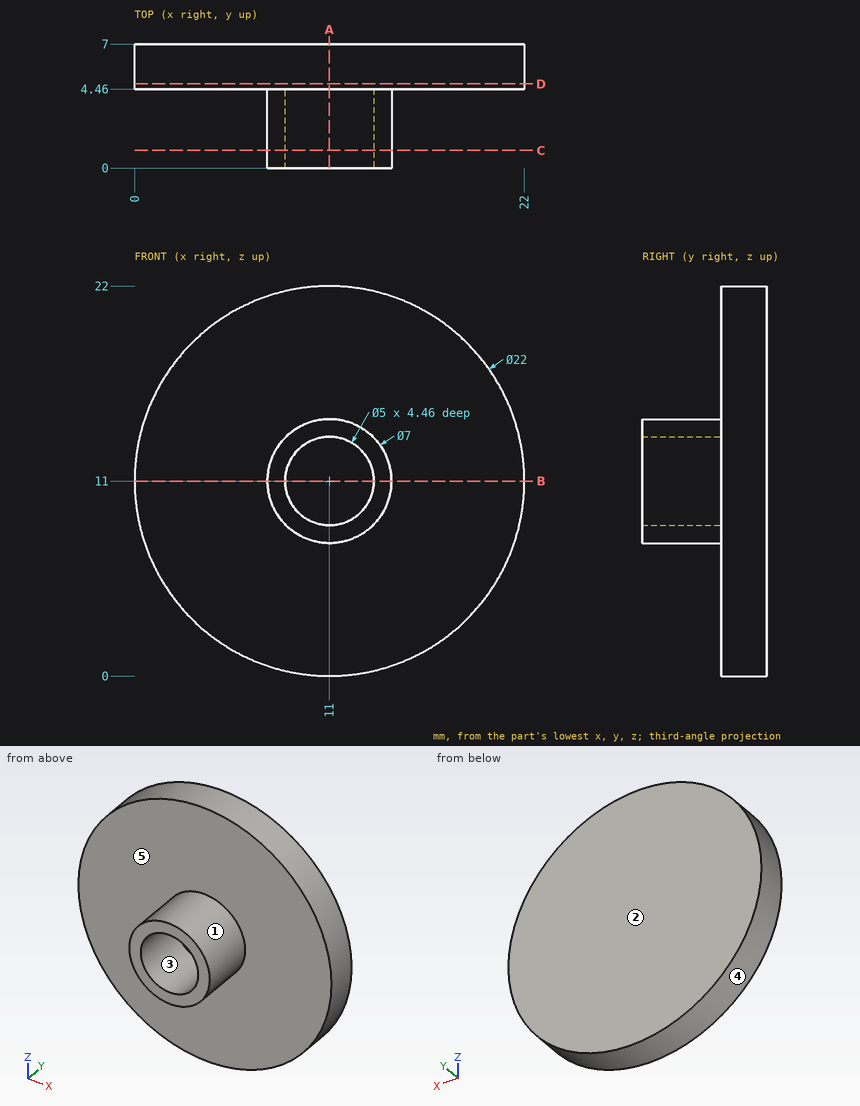
Drawing for the job (mm, zero at the part's lowest x, y, z). A direction names the side the tool comes from. Give positions to 0.01 mm unless a question says otherwise; leave off trailing zeros. Order: outer loops, then holes, each group sorted by start corner. A loop starts at its lowest first (then second) coordinate and runs counter-clockwise, first axis right, second up. Notation, with made-up numbers: (37, -23) - (56, -23) arc R6 cw to (56, -19) - close; hole circle Ø7 at (38.25, 32.5). An arc over 180 degrees is marked (long way). Write item = value, one per line. Start each with the question number.
1. Cut at D-D, the plane y = 4.75. List the corners of the cut face in (x, z), and give its area (3 significant figures).
2. Cut at B-B, the plane z = 11. List the corners of the cut face in (x, y).
3. Which spindle directions (+Z, -Z, +X, -X, +Y, -Y) get a long thin tool onto all of the face, cutting with end or side? Do the marked faces 4 and 5. Say none if no direction does.
4. Drop flat-ended pins along their axis: P1, Ø2, axis at y = 5, z = 13.5, coming from the +X side; P2, Ø4, axis at x = 12.5, y = 2, coming from the -Z side; P3, Ø5.5, axis at x = 11, z = 10.5, coming from the -Y side; P4, Ø8, axis at x = 10, z = 19, coming from the -Y side. Give the stop position or say it passes through.
5. Cut at C-C, the plane y = 1. List the corners of the cut face in (x, z), and give its area (3 significant figures).
6. Cut at A-A, the plane x = 11. List the corners of the cut face in (y, z), and give its area (3 significant figures).
7. Two-plate mould, pull along Z, no slides. Class the marked faces 1, 2 and 3: pulls with the +Z half, pulls with the -Z half, needs draft (parallel to the pull), parting line crosses it, or undercut.
8. Probe line 1 along X through (y, z) = (1.8, 11); line 2 along Y through (x, z) = (10.25, 18). List the from-to ranges inside material, lowest first.
Taken from the geometry:
q1.outline = circle Ø22 at (11, 11)
q1.area = 380 mm²
q2.outline = (0, 4.46) - (7.5, 4.46) - (7.5, 0) - (8.5, 0) - (8.5, 4.46) - (13.5, 4.46) - (13.5, 0) - (14.5, 0) - (14.5, 4.46) - (22, 4.46) - (22, 7) - (0, 7) - close
q3.face_4 = +Y, -Y
q3.face_5 = -Y
q4.P1 = 21.9
q4.P2 = 7.5
q4.P3 = 0
q4.P4 = 4.46
q5.outline = circle Ø7 at (11, 11); hole circle Ø5 at (11, 11)
q5.area = 18.8 mm²
q6.outline = (0, 7.5) - (4.46, 7.5) - (4.46, 0) - (7, 0) - (7, 22) - (4.46, 22) - (4.46, 14.5) - (0, 14.5) - (0, 13.5) - (4.46, 13.5) - (4.46, 8.5) - (0, 8.5) - close
q6.area = 64.8 mm²
q7.face_1 = parting line crosses it
q7.face_2 = needs draft
q7.face_3 = undercut
q8.line_1 = 7.5 to 8.5, 13.5 to 14.5
q8.line_2 = 4.46 to 7
